Work out the finished part from the listing and answer in its coordinate system (mm). A direction names the side the tool comes from. Coordinates: 2 decimals unless noted, no trailing zeros. Order: outer loops, then holes, each group sorted by start corner. A loop starts at its lowest first (then second) coordinate and runs counter-clockwise, first axis right, second up. Notation, with made-up numbers: M 44.5,59.25 L 75.5,59.25 A30 cw 75.5,91.25 Z; hole C 67,-38 d5. An arc over 180 degrees is marked long. Use a Markdown table: item, result.
from build123d import *

# Parameters (mm, degrees)
SKETCH1_R                  = 2.15
SKETCH1_R_2                = 2.16
BASE_FLANGE1_DEPTH         = 1.5748
SKETCHED_START             = 58.096428764
SKETCHED_BEND1_OUTLINE_W   = 50.8
SKETCHED_BEND1_OUTLINE_H   = 1.5748
SKETCHED_BEND1_DEPTH       = 24.303571236
SKETCHED_START_2           = 56.865020508
SKETCHED_BEND1_2_OUTLINE_W = 50.8
SKETCHED_BEND1_2_OUTLINE_H = 25.265020508
SKETCHED_BEND1_2_OUTLINE_R = 2.16
SKETCHED_BEND1_2_DEPTH     = 0.589203492
SKETCHED_START_3           = 55.188620508
SKETCHED_BEND1_3_OUTLINE_W = 50.8
SKETCHED_BEND1_3_OUTLINE_H = 25.265020508
SKETCHED_BEND1_3_OUTLINE_R = 2.16
SKETCHED_BEND1_3_DEPTH     = 3.2512
SKETCHED_START_4           = -12.7
SKETCHED_BEND1_4_DEPTH     = 50.8


with BuildPart() as part:
    # Base-Flange1: sheet metal written as solids
    # Sketch1 → Base-Flange1 (new body)
    with BuildSketch(Plane.XY):
        Polygon((49, 25.4), (49, 38.1), (57, 38.1), (82.4, 38.1), (82.4, -12.7), (57, -12.7), (49, -12.7), (49, 0), (0, 0), (0, 25.4), align=None)
        with Locations((3.18, 19.05)):
            Circle(SKETCH1_R, mode=Mode.SUBTRACT)
        with Locations((15.88, 19.05)):
            Circle(SKETCH1_R, mode=Mode.SUBTRACT)
        with Locations((28.58, 19.05)):
            Circle(SKETCH1_R, mode=Mode.SUBTRACT)
        with Locations((15.88, 6.35)):
            Circle(SKETCH1_R, mode=Mode.SUBTRACT)
        with Locations((28.58, 6.35)):
            Circle(SKETCH1_R, mode=Mode.SUBTRACT)
        with Locations((3.18, 6.35)):
            Circle(SKETCH1_R, mode=Mode.SUBTRACT)
        with Locations((41.28, 19.05)):
            Circle(SKETCH1_R, mode=Mode.SUBTRACT)
        with Locations((41.28, 6.35)):
            Circle(SKETCH1_R, mode=Mode.SUBTRACT)
        with Locations((64.7, 19.05)):
            Circle(SKETCH1_R_2, mode=Mode.SUBTRACT)
        with Locations((77.4, 19.05)):
            Circle(SKETCH1_R_2, mode=Mode.SUBTRACT)
        with Locations((64.7, 6.35)):
            Circle(SKETCH1_R_2, mode=Mode.SUBTRACT)
        with Locations((77.4, 6.35)):
            Circle(SKETCH1_R_2, mode=Mode.SUBTRACT)
    extrude(amount=-BASE_FLANGE1_DEPTH)

    # Sketched Bend1: read off the stored shape, not the designer's step
    # Sketched Bend1 outline → Sketched Bend1 (cut)
    with BuildSketch(Plane.YZ.offset(SKETCHED_START)):
        with Locations((12.7, -0.7874)):
            Rectangle(SKETCHED_BEND1_OUTLINE_W, SKETCHED_BEND1_OUTLINE_H)
    extrude(amount=SKETCHED_BEND1_DEPTH, mode=Mode.SUBTRACT)

    # Sketched Bend1 2 outline → Sketched Bend1 2 (add)
    with BuildSketch(Plane.YZ.offset(SKETCHED_START_2)):
        with Locations((12.7, -14.207310254)):
            Rectangle(SKETCHED_BEND1_2_OUTLINE_W, SKETCHED_BEND1_2_OUTLINE_H)
        with Locations((6.35, -21.839820508)):
            Circle(SKETCHED_BEND1_2_OUTLINE_R, mode=Mode.SUBTRACT)
        with Locations((19.05, -21.839820508)):
            Circle(SKETCHED_BEND1_2_OUTLINE_R, mode=Mode.SUBTRACT)
        with Locations((6.35, -9.139820508)):
            Circle(SKETCHED_BEND1_2_OUTLINE_R, mode=Mode.SUBTRACT)
        with Locations((19.05, -9.139820508)):
            Circle(SKETCHED_BEND1_2_OUTLINE_R, mode=Mode.SUBTRACT)
    extrude(amount=SKETCHED_BEND1_2_DEPTH)

    # Sketched Bend1 3 outline → Sketched Bend1 3 (add)
    with BuildSketch(Plane.YZ.offset(SKETCHED_START_3)):
        with Locations((12.7, -14.207310254)):
            Rectangle(SKETCHED_BEND1_3_OUTLINE_W, SKETCHED_BEND1_3_OUTLINE_H)
        with Locations((6.35, -21.839820508)):
            Circle(SKETCHED_BEND1_3_OUTLINE_R, mode=Mode.SUBTRACT)
        with Locations((19.05, -21.839820508)):
            Circle(SKETCHED_BEND1_3_OUTLINE_R, mode=Mode.SUBTRACT)
        with Locations((6.35, -9.139820508)):
            Circle(SKETCHED_BEND1_3_OUTLINE_R, mode=Mode.SUBTRACT)
        with Locations((19.05, -9.139820508)):
            Circle(SKETCHED_BEND1_3_OUTLINE_R, mode=Mode.SUBTRACT)
    extrude(amount=SKETCHED_BEND1_3_DEPTH)

    # Sketched Bend1 4 outline → Sketched Bend1 4 (cut)
    with BuildSketch(Plane(origin=(0, 0, 0), x_dir=(1, 0, 0), z_dir=(0, 1, 0)).offset(SKETCHED_START_4)):
        with BuildLine():
            Line((56.865020508, 3.2512), (56.865020508, 26.839820508))
            Line((56.865020508, 26.839820508), (55.188620508, 26.839820508))
            Line((55.188620508, 26.839820508), (55.188620508, 1.5748))
            ThreePointArc((55.188620508, 1.5748), (56.374014316, 2.065806192), (56.865020508, 3.2512))
        make_face()
        with BuildLine():
            Line((58.439820508, 1.5748), (58.439820508, 3.2512))
            ThreePointArc((58.439820508, 3.2512), (57.487566075, 0.952254433), (55.188620508, 0))
            Line((55.188620508, 0), (58.096428764, 0))
            Line((58.096428764, 0), (58.096428764, 1.5748))
            Line((58.096428764, 1.5748), (58.439820508, 1.5748))
        make_face()
    extrude(amount=SKETCHED_BEND1_4_DEPTH, mode=Mode.SUBTRACT)


solid = part.part
1. For faces 4 (the face through (24, 25.4, -1)), 5 (the face through (49, -6, -1)), 6 (the face through (34, 13, -1.575)), determine the directions among +Z, -Z, +X, -X, +Y, -Y from which every point of the face is accessible in a straight line to the end or side of a thin tool.
Answers below:
| item | result |
|---|---|
| face 4 | +Z, -Z, -X, +Y |
| face 5 | +Z, -Z, -X, -Y |
| face 6 | -Z, -X, +Y, -Y |
2. Section C-C on y = 16 is taken. Determine the outline of the cut face in (x, z), then the cut area to 3 significant figures.
Answers below:
| item | result |
|---|---|
| outline | M 0,-1.57 L 55.19,-1.57 A1.68 cw 56.87,-3.25 L 56.87,-26.84 L 58.44,-26.84 L 58.44,-3.25 A3.25 ccw 55.19,0 L 0,0 Z |
| area | 130 mm² |
3. Flat-ended cylindrical pins translate along their axes: P1, Ø3.5, axis at x = 28.58, y = 19.05, coming from the +Z side; P2, Ø3, axis at y = -7, z = -17.5, coming from the -X side (3 decimals); P3, Ø0.8, axis at y = -7, z = -0.5, coming from the -X side; P4, Ø5, axis at x = 41.28, y = 19.05, coming from the -Z side. Find the tip coordinate at first contact, or state that the pin passes through.
Answers below:
| item | result |
|---|---|
| P1 | through |
| P2 | x = 56.865 |
| P3 | x = 49 |
| P4 | z = -1.57 |
4. Section A-A on x = 28.58 is taken. Determine the outline of the cut face in (y, z), then the cut area to 3 significant figures.
Answers below:
| item | result |
|---|---|
| outline | M 0,-1.57 L 4.2,-1.57 L 4.2,0 L 0,0 Z; M 8.5,-1.57 L 16.9,-1.57 L 16.9,0 L 8.5,0 Z; M 21.2,-1.57 L 25.4,-1.57 L 25.4,0 L 21.2,0 Z |
| area | 26.5 mm² |
5. Section D-D on x = 45 is taken. Determine the outline of the cut face in (y, z), then the cut area to 3 significant figures.
Answers below:
| item | result |
|---|---|
| outline | M 0,-1.57 L 25.4,-1.57 L 25.4,0 L 0,0 Z |
| area | 40.0 mm² |
6. For a pull along X with two mould halves and no side action, classify faces 1 (the face through (57.2, -12.7, -9.5)), 2 (the face through (49, 32, -1)), 3 (the face through (26.43, 19.14, -0.78)) as +X half, -X half, draft (parallel to the pull), parting line (faces both ways), or undercut.
Answers below:
| item | result |
|---|---|
| face 1 | draft |
| face 2 | -X half |
| face 3 | undercut |
7. Section B-B on y = 6.35 is taken. Give the number of separate pieces and of enclosed holes in the cut face, then the cut area to 3 significant figures.
Answers below:
| item | result |
|---|---|
| separate pieces | 7 |
| enclosed holes | 0 |
| area | 89.5 mm² |
8. Find the intervals of material crossed by probe 1 along Y at (x, z) = (15.88, -0.8); probe 2 along Z at (x, y) = (57, 6); probe 3 along X at (y, z) = (18, -5.5), in increasing order.
Answers below:
| item | result |
|---|---|
| probe 1 | 0 to 4.2, 8.5 to 16.9, 21.2 to 25.4 |
| probe 2 | -26.84 to -23.97, -19.71 to -11.27, -7.01 to -0.55 |
| probe 3 | 56.87 to 58.44 |
